```python
from build123d import *

# Parameters (mm, degrees)
MODEL_R         = 1.5
MODEL_R_2       = 9
EXTRUDE_1_DEPTH = 2


with BuildPart() as part:
    # Model → 凸台-拉伸1 (new body)
    with BuildSketch(Plane.XY):
        with BuildLine():
            Line((0.203212392, 23.351643478), (-7.191181553, 14.724665579))
            ThreePointArc((-7.191181553, 14.724665579), (-8.556294423, 14.032124893), (-10.011275206, 14.507705245))
            Line((-10.011275206, 14.507705245), (-13.011488382, 17.079261403))
            ThreePointArc((-13.011488382, 17.079261403), (-15.873946091, 18.033792422), (-18.588835359, 16.71691359))
            ThreePointArc((-18.588835359, 16.71691359), (8.377839615, -23.554443389), (3.857459976, 24.700607331))
            ThreePointArc((3.857459976, 24.700607331), (1.855038258, 24.500995075), (0.203212392, 23.351643478))
        make_face()
        with Locations((-18, 0)):
            Circle(MODEL_R, mode=Mode.SUBTRACT)
        with Locations((18, 0)):
            Circle(MODEL_R, mode=Mode.SUBTRACT)
        Circle(MODEL_R_2, mode=Mode.SUBTRACT)
        with Locations((0, 18)):
            Circle(MODEL_R, mode=Mode.SUBTRACT)
        with Locations((0, -18)):
            Circle(MODEL_R, mode=Mode.SUBTRACT)
    extrude(amount=EXTRUDE_1_DEPTH)


solid = part.part
```
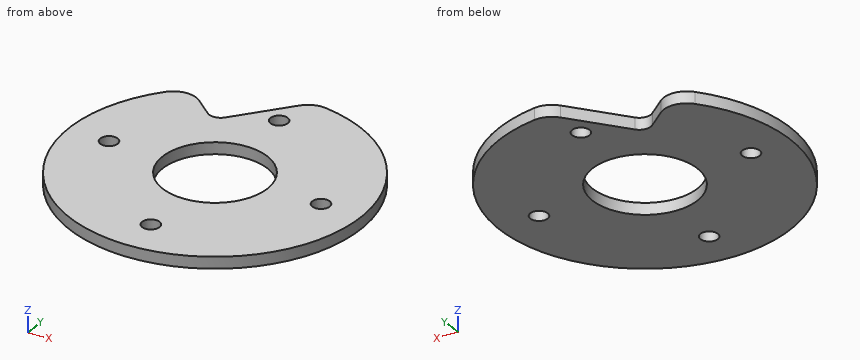
The listing builds one solid part. Answer for the finished solid, in the listing's coordinates (mm). Coordinates: 2 decimals unless noted, no trailing zeros. Write each loop counter-clockwise with the first axis right and the second up, starting at its lowest first coordinate (ties: lowest second). Pieces come first, ordered by that corner, then holes.
Q1. Section C-C, the plane z = 0.75 is taken. Write down the section's boundary in (x, y).
Returned:
outline: (-18.59, 16.72) arc R25 ccw (long way) to (3.86, 24.7) arc R4 ccw to (0.2, 23.35) - (-7.19, 14.72) arc R2 cw to (-10.01, 14.51) - (-13.01, 17.08) arc R4 ccw to start; hole circle Ø3 at (-18, 0); hole circle Ø18 at (0, 0); hole circle Ø3 at (0, -18); hole circle Ø3 at (0, 18); hole circle Ø3 at (18, 0)
Q2. Section B-B, the plane x = 18 is taken. Write down the section's boundary in (y, z).
Returned:
outline: (-17.35, 0) - (-1.5, 0) - (-1.5, 2) - (-17.35, 2) - close; (1.5, 0) - (17.35, 0) - (17.35, 2) - (1.5, 2) - close
Q3. Find the intervals of material crossed by line 1 along Y through (x, z) = (0, 1); line 2 along Y through (x, z) = (2.5, 1.4); line 3 along Y through (x, z) = (4, 1.75), in increasing order.
Returned:
line 1: y = -25 to -19.5, -16.5 to -9, 9 to 16.5, 19.5 to 23.11
line 2: y = -24.87 to -8.65, 8.65 to 24.68
line 3: y = -24.68 to -8.06, 8.06 to 24.68
Q4. Given P1, Ø1.8, axis at x = 0, y = -18, coming from the -Z side; P2, Ø1, axis at y = -10, z = 0.5, coming from the +X side, each flat-ended and moving along its own axis, determine where each tip first touches the part or whether it passes through.
Returned:
P1: passes through
P2: stops at x = 23.12
Q5. Section A-A, the plane y = 0 is taken. Write down the section's boundary in (x, z).
Returned:
outline: (-25, 0) - (-19.5, 0) - (-19.5, 2) - (-25, 2) - close; (-16.5, 0) - (-9, 0) - (-9, 2) - (-16.5, 2) - close; (9, 0) - (16.5, 0) - (16.5, 2) - (9, 2) - close; (19.5, 0) - (25, 0) - (25, 2) - (19.5, 2) - close
